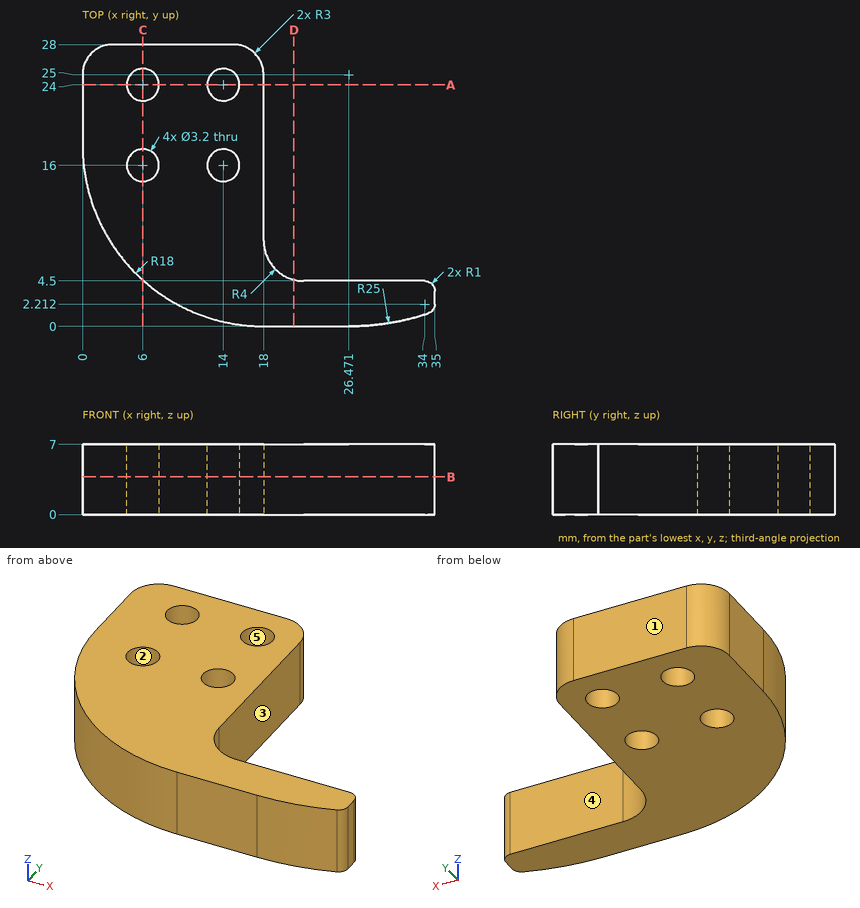
Design review of the part shown in the three views and the two pictorial views. Dimensions are in mm from the part's minimum x, y and z. A direction names the side the tool comes from. Coordinates: 2 decimals unless noted, no trailing zeros. Loops run counter-clockwise (first coordinate to the right, second up) from the corner with the lowest first, then second, coordinate; pieces in that order, holes last.
Q1. We need section C-C on x = 6. State the section outline as (y, z) points.
Reported:
outline: (4.58, 0) - (14.4, 0) - (14.4, 7) - (4.58, 7) - close; (17.6, 0) - (22.4, 0) - (22.4, 7) - (17.6, 7) - close; (25.6, 0) - (28, 0) - (28, 7) - (25.6, 7) - close
Q2. We need section B-B on z = 3.75. State the section outline as (x, y) points, and give its area (3 significant figures).
Reported:
outline: (0, 18) arc R18 ccw to (18, 0) - (26.47, 0) arc R25 ccw to (34.31, 1.26) arc R1 ccw to (35, 2.21) - (35, 3.5) arc R1 ccw to (34, 4.5) - (22, 4.5) arc R4 cw to (18, 8.5) - (18, 25) arc R3 ccw to (15, 28) - (3, 28) arc R3 ccw to (0, 25) - close; hole circle Ø3.2 at (6, 16); hole circle Ø3.2 at (6, 24); hole circle Ø3.2 at (14, 16); hole circle Ø3.2 at (14, 24)
area: 474 mm2
Q3. To check wall thickness, follow line 1 (X direction, y = 24.5, z = 2.5); line 2 (Y direction, x = 14, z = 2); line 3 (Y direction, x = 15, z = 3.75). State the ranges of each line that lie inside material, in increasing order.
Reported:
line 1: x = 0 to 4.48, 7.52 to 12.48, 15.52 to 18
line 2: y = 0.45 to 14.4, 17.6 to 22.4, 25.6 to 28
line 3: y = 0.25 to 14.75, 17.25 to 22.75, 25.25 to 28
Q4. The part is to be moulded in two halves that separate along Y. For the marked faces 1, 2 and 3, say which applies: +Y half, -Y half, draft (parallel to the pull), parting line (faces both ways), or undercut.
Reported:
face 1: +Y half
face 2: undercut
face 3: draft
Q5. Tool access review of the marked faces 4 and 5: name each direction out of +Z, -Z, +X, -X, +Y, -Y from which nothing blocks a thin tool from reaching the whole face with its end or side.
Reported:
face 4: +Z, -Z, +X, +Y
face 5: +Z, -Z
Q6. We need section D-D on x = 21. State the section outline as (y, z) points, and give its area (3 significant figures).
Reported:
outline: (0, 0) - (4.63, 0) - (4.63, 7) - (0, 7) - close
area: 32.4 mm2
Q7. For pin 1 (2 mm diameter, centred on y = 17.5, z = 4, fed in from +X); pin 2 (1 mm diameter, centred on y = 10.5, z = 3, fed in from -X); pin 3 (1.5 mm diameter, centred on x = 29, z = 1.5, fed in from +Y), all flat-tipped, find the tip position at first contact; note any pin that passes through.
Reported:
pin 1: stops at x = 18
pin 2: stops at x = 1.42
pin 3: stops at y = 4.5
Q8. We need section A-A on y = 24. State the section outline as (x, z) points, and give its area (3 significant figures).
Reported:
outline: (0, 0) - (4.4, 0) - (4.4, 7) - (0, 7) - close; (7.6, 0) - (12.4, 0) - (12.4, 7) - (7.6, 7) - close; (15.6, 0) - (18, 0) - (18, 7) - (15.6, 7) - close
area: 81.2 mm2
